from build123d import *

# Parameters (mm, degrees)
F1_DEPTH = 50
F2_R     = 3.5
F3_DEPTH = 25
F4_R     = 2.5
F5_DEPTH = 40.001


with BuildPart() as f1:
    # F0 (on Top) → F1 (new body)
    with BuildSketch(Plane.XY):
        Polygon((0, 48), (0, 0), (40, 0), (40, 48), (35, 48), (35, 10), (5, 10), (5, 48), align=None)
    extrude(amount=F1_DEPTH)

    # F2 (on face) → F3 (cut)
    with BuildSketch(Plane.XZ):
        with Locations((20, 25)):
            Circle(F2_R)
    extrude(amount=-F3_DEPTH, mode=Mode.SUBTRACT)

    # F4 (on face) → F5 (cut, through all)
    with BuildSketch(Plane.YZ.offset(40)):
        with Locations((35, 25)):
            Circle(F4_R)
    extrude(amount=-F5_DEPTH, mode=Mode.SUBTRACT)


solid = f1.part
Read the model definition and answer for the solid it produces. Units are mm, in the model's axes. A direction names the side the tool comes from. Give positions to 0.01 mm unless a question says otherwise; leave off trailing zeros. Write each loop counter-clockwise with the first axis right and the second up, starting at its lowest first coordinate (ties: lowest second). Pieces come first, ordered by that corner, then holes. Notation, with made-up numbers: M 85.5,11 L 99.5,11 A21 ccw 99.5,46 Z; hole C 85,69.25 d3. An arc over 180 degrees is marked long. One line per item, written item: value. Start each with the question number.
(1) Determine the mould class of faces 1 (the cylindrical face through (2.53, 36.34, 27.11)), 2 (the flat face through (5, 29, 25)), 3 (the flat face through (0, 24, 25)), 4 (the flat face through (40, 24, 25)) for opening direction X: pulls with the +X half, pulls with the -X half, needs draft (parallel to the pull), parting line crosses it, or undercut.
(2) Find the intervals of material crossed by line 1 (X direction, y = 45, z = 28.5); line 2 (Z direction, x = 20, y = 4); line 3 (Z direction, x = 1, y = 35), in increasing order.
(3) A tool of negligible diameter and unlimited length cuts with its end or side. For faces 5 (the flat face through (35, 29, 25)), 6 (the cylindrical face through (23.34, 4.93, 26.05)), from which of +Z, -Z, +X, -X, +Y, -Y can it reach the whole face along a straight path? Write none if from no direction.
(4) Find section D-D (y = 12). Determine the outline of the cut face in (x, z), plus the area to 3 significant figures.
(5) Find section A-A (x = 20). Determine the outline of the cut face in (y, z), plus the area to 3 significant figures.
(6) Find section C-C (y = 35). Determine the outline of the cut face in (x, z), plus the area to 3 significant figures.
(7) Find section B-B (z = 25). Determine the outline of the cut face in (x, y).
(8) Flat-ended cylindrical pins translate along their axes: pin 1 Ø4.5 at (y, z) = (35, 25) entering from -X; pin 2 Ø15 at (x, z) = (19.5, 28) entering from +Y. Find the tip coordinate at first contact, or state that the pin passes through.
Results below:
1. face 1: needs draft
1. face 2: undercut
1. face 3: pulls with the -X half
1. face 4: pulls with the +X half
2. line 1: x = 0 to 5, 35 to 40
2. line 2: z = 0 to 21.5, 28.5 to 50
2. line 3: z = 0 to 22.5, 27.5 to 50
3. face 5: +Z, -Z, +Y
3. face 6: +Y, -Y
4. outline: M 0,0 L 5,0 L 5,50 L 0,50 Z; M 35,0 L 40,0 L 40,50 L 35,50 Z
4. area: 500 mm^2
5. outline: M 0,0 L 10,0 L 10,21.5 L 0,21.5 Z; M 0,28.5 L 10,28.5 L 10,50 L 0,50 Z
5. area: 430 mm^2
6. outline: M 0,0 L 5,0 L 5,22.5 L 0,22.5 Z; M 0,27.5 L 5,27.5 L 5,50 L 0,50 Z; M 35,0 L 40,0 L 40,22.5 L 35,22.5 Z; M 35,27.5 L 40,27.5 L 40,50 L 35,50 Z
6. area: 450 mm^2
7. outline: M 0,0 L 16.5,0 L 16.5,10 L 5,10 L 5,32.5 L 0,32.5 Z; M 0,37.5 L 5,37.5 L 5,48 L 0,48 Z; M 23.5,0 L 40,0 L 40,32.5 L 35,32.5 L 35,10 L 23.5,10 Z; M 35,37.5 L 40,37.5 L 40,48 L 35,48 Z
8. pin 1: passes through
8. pin 2: stops at y = 10
